```python
from build123d import *

# Parameters (mm, degrees)
SKETCH1_W           = 160
SKETCH1_H           = 160
BOSS_EXTRUDE1_DEPTH = 9
SKETCH2_W           = 9
SKETCH2_H           = 15
SKETCH2_H_2         = 9
BOSS_EXTRUDE2_DEPTH = 9
SKETCH3_R           = 1.7
SKETCH3_W           = 9
SKETCH3_H           = 15
CUT_EXTRUDE1_DEPTH  = 121.008333044
CUT_EXTRUDE2_DEPTH  = 121.008333044
SKETCH5_R           = 9.5
SKETCH5_R_2         = 2.75
CUT_EXTRUDE3_DEPTH  = 121.008333044


with BuildPart() as part:
    # Sketch1 → Boss-Extrude1 (new body)
    with BuildSketch(Plane(origin=(0, 0, 0), x_dir=(1, 0, 0), z_dir=(0, 1, 0))):
        Rectangle(SKETCH1_W, SKETCH1_H)
    extrude(amount=BOSS_EXTRUDE1_DEPTH)

    # Sketch2 → Boss-Extrude2 (add)
    with BuildSketch(Plane(origin=(0, 9, 0), x_dir=(1, 0, 0), z_dir=(0, 1, 0))):
        with Locations((-84.5, 0)):
            Rectangle(SKETCH2_W, SKETCH2_H)
        with Locations((-84.5, 43.75)):
            Rectangle(SKETCH2_W, SKETCH2_H)
        with Locations((-84.5, -43.75)):
            Rectangle(SKETCH2_W, SKETCH2_H)
        with Locations((-84.5, 75.5)):
            Rectangle(SKETCH2_W, SKETCH2_H_2)
        with Locations((-84.5, -75.5)):
            Rectangle(SKETCH2_W, SKETCH2_H_2)
    extrude(amount=-BOSS_EXTRUDE2_DEPTH)

    # Sketch3 → Cut-Extrude1 (cut, through all)
    with BuildSketch(Plane(origin=(0, 9, 0), x_dir=(1, 0, 0), z_dir=(0, 1, 0))):
        with Locations(Location((70.5, 21.875, 0), (0, 0, 270))):
            Circle(SKETCH3_R)
        with Locations(Location((70.5, -21.875, 0), (0, 0, 270))):
            Circle(SKETCH3_R)
        with Locations((70.5, 43.75)):
            Rectangle(SKETCH3_W, SKETCH3_H)
        with Locations((70.5, 0)):
            Rectangle(SKETCH3_W, SKETCH3_H)
        with Locations((70.5, -43.75)):
            Rectangle(SKETCH3_W, SKETCH3_H)
    extrude(amount=-CUT_EXTRUDE1_DEPTH, mode=Mode.SUBTRACT)

    # Sketch4 → Cut-Extrude2 (cut, through all)
    with BuildSketch(Plane(origin=(0, 9, 0), x_dir=(1, 0, 0), z_dir=(0, 1, 0))):
        Polygon((-80, 23.575), (-76.2, 23.575), (-76.2, 24.625), (-74, 24.625), (-74, 23.575), (-71, 23.575), (-71, 20.175), (-74, 20.175), (-74, 19.125), (-76.2, 19.125), (-76.2, 20.175), (-80, 20.175), align=None)
        Polygon((-80, -23.575), (-80, -20.175), (-76.2, -20.175), (-76.2, -19.125), (-74, -19.125), (-74, -20.175), (-71, -20.175), (-71, -23.575), (-74, -23.575), (-74, -24.625), (-76.2, -24.625), (-76.2, -23.575), align=None)
    extrude(amount=-CUT_EXTRUDE2_DEPTH, mode=Mode.SUBTRACT)

    # Sketch5 → Cut-Extrude3 (cut, through all)
    with BuildSketch(Plane(origin=(0, 9, 0), x_dir=(1, 0, 0), z_dir=(0, 1, 0))):
        with Locations(Location((0, 0, 0), (0, 0, 270))):
            Circle(SKETCH5_R)
        with Locations(Location((-20, 40.25, 0), (0, 0, 270))):
            Circle(SKETCH5_R_2)
        with Locations(Location((20, 40.25, 0), (0, 0, 270))):
            Circle(SKETCH5_R_2)
        with Locations(Location((20, -40.25, 0), (0, 0, 270))):
            Circle(SKETCH5_R_2)
        with Locations(Location((-20, -40.25, 0), (0, 0, 270))):
            Circle(SKETCH5_R_2)
    extrude(amount=-CUT_EXTRUDE3_DEPTH, mode=Mode.SUBTRACT)


solid = part.part
```
The model under review builds one solid part; all positions refer to its coordinate system, in mm. A direction names the side the tool comes from. Round coordinates to 2 decimals unless told otherwise and drop trailing zeros. Loops run counter-clockwise (first coordinate to the right, second up) from the corner with the lowest first, then second, coordinate; pieces in that order, holes last. Notation, with made-up numbers: (13.25, 86.25) - (71.25, 86.25) arc R13 cw to (71.25, 95.25) - close; hole circle Ø11 at (-38.75, -29.5). An arc over 180 degrees is marked (long way). Use a Markdown table: item, result. Add a question column.
Q1. Add section B-B (z = -5.5). State the section outline as (x, y) points.
Q2. Insertion check: pin 1 Ø5 at (y, z) = (3, 56) entering from -X; pin 2 Ø2.5 at (y, z) = (5, 21.5) entering from -X. Each pin has a flat end and moves straight along its axis. Give the tip position at first contact, or say it passes through.
Q3. The part is to be moulded in two halves that separate along X. For faces 1 (the face through (-85, 5, -7.5)), 2 (the face through (75, 5, 0)), 3 (the face through (66, 5, 44)), say which applies: pulls with the +X half, pulls with the -X half, needs draft (parallel to the pull), parting line crosses it, or undercut.
Q4. Add section C-C (y = 5.25). State how many separate pieces and enclosed holes the cut face has, plus the area to 3 significant figures.
Q5. Add section D-D (z = 58.5). State the section outline as (x, y) points, plus the area to 3 significant figures.
Q6. Add section A-A (z = 40.25). State the section outline as (x, y) points.
Q7. For probe 1 along X at (y, z) = (4, -40.25); probe 2 along X at (y, z) = (7, 0); probe 3 along X at (y, z) = (3.5, -51), list the stretches that pass through material, from the lowest coordinate up.
Q8. Machinability: for faces 4 (the face through (-85, 5, 7.5)), 5 (the face through (13, 0, -1)), 6 (the face through (75, 5, -44)), which of the approach directions +Z, -Z, +X, -X, +Y, -Y give a long, thin tool a straight path to every point of the face, cutting with its end or side? Answer none if there is none.
Worked answers:
| question | item | result |
|---|---|---|
| 1 | outline | (-89, 0) - (-7.75, 0) - (-7.75, 9) - (-89, 9) - close; (7.75, 0) - (66, 0) - (66, 9) - (7.75, 9) - close; (75, 0) - (80, 0) - (80, 9) - (75, 9) - close |
| 2 | pin 1 | x = -80 |
| 2 | pin 2 | x = -71 |
| 3 | face 1 | needs draft |
| 3 | face 2 | undercut |
| 3 | face 3 | undercut |
| 4 | separate pieces | 1 |
| 4 | enclosed holes | 10 |
| 4 | area | 25,300 mm² |
| 5 | outline | (-80, 0) - (80, 0) - (80, 9) - (-80, 9) - close |
| 5 | area | 1,440 mm² |
| 6 | outline | (-89, 0) - (-22.75, 0) - (-22.75, 9) - (-89, 9) - close; (-17.25, 0) - (17.25, 0) - (17.25, 9) - (-17.25, 9) - close; (22.75, 0) - (66, 0) - (66, 9) - (22.75, 9) - close; (75, 0) - (80, 0) - (80, 9) - (75, 9) - close |
| 7 | probe 1 | -89 to -22.75, -17.25 to 17.25, 22.75 to 66, 75 to 80 |
| 7 | probe 2 | -89 to -9.5, 9.5 to 66, 75 to 80 |
| 7 | probe 3 | -89 to 66, 75 to 80 |
| 8 | face 4 | -X, +Y, -Y |
| 8 | face 5 | +Z, -Z, +X, -X, -Y |
| 8 | face 6 | +Y, -Y |
